Geometry: final body of the model. Coordinates: model frame, mm. Face numbers are marked on the shaded views. A direction names the side the tool comes from. Give positions to 0.01 mm unless a question says otherwise; leave off trailing zeros. Loops run counter-clockwise (first coordinate to the right, second up) from the corner with the lowest first, then second, coordinate; pieces in that order, holes last.
1. Section C-C, the plane x = 23.5. Output: boundary loops of the cut face in (y, z), then the cut area to 3 significant figures.
2. Draft query along X for the marked faces 4, 5, 6 and 7. Return one class per face: +X half, -X half, draft (parallel to the pull), parting line (faces both ways), or undercut.
3. Material intervals for line 1 along Z through (x, y) = (45, 16); line 2 along X through (y, z) = (13.25, 22.5); line 3 along Z through (x, y) = (15, 16.75), sorted ascending.
4. Access query for the marked faces 1, 2 and 3. Directions: +Z, -Z, +X, -X, +Y, -Y. A direction counts if a zero-diameter tool reaches every point of the face in a straight line with its end or side. Return the directions, or none.
5. Section A-A, the plane y = 7.75. Output: boundary loops of the cut face in (x, z).
6. Section B-B, the plane y = 11.5. Output: boundary loops of the cut face in (x, z).
7. Section D-D, the plane z = 7.5. Output: boundary loops of the cut face in (x, y).
8. First-contact query: P1, Ø2.5, axis at x = 33, z = 33.5, coming from the -Y side; P2, Ø3, axis at x = 45, z = 0, coming from the +Y side; P3, Ø1.5, axis at x = 9, z = 4.5, coming from the +Y side. Flat tips, straight axial feed; report the tip coordinate or a pass-through.
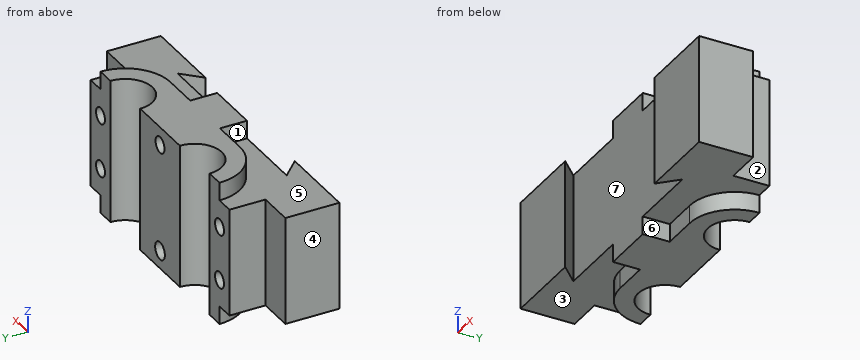
from build123d import *

# Parameters (mm, degrees)
BOSS_EXTRUDE2_DEPTH = 30
BOSS_EXTRUDE3_DEPTH = 5
BOSS_EXTRUDE4_DEPTH = 5
SKETCH5_R           = 2.25
SKETCH5_R_2         = 2.445661488
CUT_EXTRUDE2_DEPTH  = 15


with BuildPart() as part:
    # Sketch1 → Boss-Extrude2 (new body)
    with BuildSketch(Plane.XY):
        with BuildLine():
            Line((0, 0), (0, 15))
            Line((0, 15), (10, 15))
            Line((10, 15), (10, 25))
            Line((10, 25), (20, 25))
            ThreePointArc((20, 25), (27.5, 17.5), (35, 25))
            Line((35, 25), (55, 25))
            ThreePointArc((55, 25), (62.5, 17.5), (70, 25))
            Line((70, 25), (80, 25))
            Line((80, 25), (80, 15))
            Line((80, 15), (90, 15))
            Line((90, 15), (90, 0))
            Line((90, 0), (67.5, 0))
            Line((67.5, 0), (72.5, 5))
            Line((72.5, 5), (17.5, 5))
            Line((17.5, 5), (22.5, 0))
            Line((22.5, 0), (0, 0))
        make_face()
    extrude(amount=BOSS_EXTRUDE2_DEPTH)

    # Sketch3 → Boss-Extrude3 (add)
    with BuildSketch(Plane.XY.offset(30)):
        with BuildLine():
            Line((70, 25), (75, 25))
            ThreePointArc((75, 25), (71.338834765, 16.161165235), (62.5, 12.5))
            Line((62.5, 12.5), (52.5, 12.5))
            Line((52.5, 12.5), (52.5, 5))
            Line((52.5, 5), (37.5, 5))
            Line((37.5, 5), (37.5, 12.5))
            Line((37.5, 12.5), (27.5, 12.5))
            ThreePointArc((27.5, 12.5), (18.661165235, 16.161165235), (15, 25))
            Line((15, 25), (20, 25))
            ThreePointArc((20, 25), (27.5, 17.5), (35, 25))
            Line((35, 25), (55, 25))
            ThreePointArc((55, 25), (62.5, 17.5), (70, 25))
        make_face()
    extrude(amount=BOSS_EXTRUDE3_DEPTH)

    # Sketch4 → Boss-Extrude4 (add)
    with BuildSketch(Plane(origin=(0, 0, 0), x_dir=(-1, 0, 0), z_dir=(0, 0, -1))):
        with BuildLine():
            Line((-62.5, 12.5), (-52.5, 12.5))
            Line((-52.5, 12.5), (-52.5, 5))
            Line((-52.5, 5), (-37.5, 5))
            Line((-37.5, 5), (-37.5, 12.5))
            Line((-37.5, 12.5), (-27.5, 12.5))
            ThreePointArc((-27.5, 12.5), (-18.661165235, 16.161165235), (-15, 25))
            Line((-15, 25), (-20, 25))
            ThreePointArc((-20, 25), (-27.5, 17.5), (-35, 25))
            Line((-35, 25), (-55, 25))
            ThreePointArc((-55, 25), (-62.5, 17.5), (-70, 25))
            Line((-70, 25), (-75, 25))
            ThreePointArc((-75, 25), (-71.338834765, 16.161165235), (-62.5, 12.5))
        make_face()
    extrude(amount=BOSS_EXTRUDE4_DEPTH)

    # Sketch5 → Cut-Extrude2 (cut)
    with BuildSketch(Plane(origin=(0, 25, 0), x_dir=(1, 0, 0), z_dir=(0, 1, 0))):
        with Locations((75, -7.5)):
            Circle(SKETCH5_R)
        with Locations((75, -22.5)):
            Circle(SKETCH5_R)
        with Locations((15, -22.5)):
            Circle(SKETCH5_R)
        with Locations((15, -7.5)):
            Circle(SKETCH5_R)
        with Locations((45, 0)):
            Circle(SKETCH5_R_2)
        with Locations((45, -30)):
            Circle(SKETCH5_R)
    extrude(amount=-CUT_EXTRUDE2_DEPTH, mode=Mode.SUBTRACT)


solid = part.part
Answers below:
1. outline: (5, 0) - (13.16, 0) - (13.16, -5) - (18.66, -5) - (18.66, 35) - (13.16, 35) - (13.16, 30) - (5, 30) - close
1. area: 465 mm2
2. face 4: -X half
2. face 5: draft
2. face 6: +X half
2. face 7: undercut
3. line 1: z = -5 to -2.45, 2.45 to 27.75, 32.25 to 35
3. line 2: x = 0 to 12.75, 17.25 to 72.75, 77.25 to 90
3. line 3: z = 0 to 5.25, 9.75 to 20.25, 24.75 to 30
4. face 1: +Z, -X, -Y
4. face 2: +Z, -Z, +X, +Y
4. face 3: -Z, -X, -Y
5. outline: (0, 0) - (37.5, 0) - (37.5, -5) - (52.5, -5) - (52.5, 0) - (90, 0) - (90, 30) - (52.5, 30) - (52.5, 35) - (37.5, 35) - (37.5, 30) - (0, 30) - close
6. outline: (0, 0) - (37.5, 0) - (37.5, -5) - (52.5, -5) - (52.5, 0) - (90, 0) - (90, 30) - (52.5, 30) - (52.5, 35) - (37.5, 35) - (37.5, 30) - (0, 30) - close; hole circle Ø4.5 at (15, 7.5); hole circle Ø4.5 at (15, 22.5); hole circle Ø4.89 at (45, 0); hole circle Ø4.5 at (45, 30); hole circle Ø4.5 at (75, 7.5); hole circle Ø4.5 at (75, 22.5)
7. outline: (0, 0) - (22.5, 0) - (17.5, 5) - (72.5, 5) - (67.5, 0) - (90, 0) - (90, 15) - (80, 15) - (80, 25) - (77.25, 25) - (77.25, 10) - (72.75, 10) - (72.75, 25) - (70, 25) arc R7.5 cw to (55, 25) - (35, 25) arc R7.5 cw to (20, 25) - (17.25, 25) - (17.25, 10) - (12.75, 10) - (12.75, 25) - (10, 25) - (10, 15) - (0, 15) - close
8. P1: stops at y = 12.5
8. P2: stops at y = 10
8. P3: stops at y = 15
